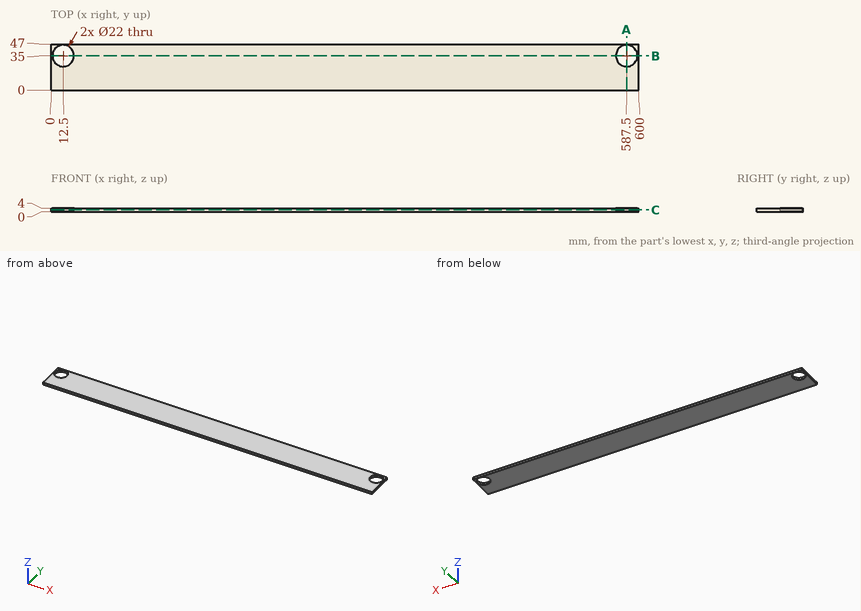
Can you work these out from the drawing? Everything is in mm from the part's minimum corner. Coordinates: 2 decimals unless noted, no trailing zeros. Loops run counter-clockwise (first coordinate to the right, second up) from the corner with the lowest first, then second, coordinate; pieces in that order, holes last.
1. Imagine slicing it at B-B, the plane y = 35. Please give me the cut outline in (x, z).
2. Imagine slicing it at A-A, the plane x = 587.5. Please give me the cut outline in (y, z), and give its area (3 significant figures).
3. Imagine slicing it at C-C, the plane z = 2.2. Please give me the cut outline in (x, y), and give its area (3 significant figures).
4. I need wall thicknesses on L1, parallel to X at y = 35.5, z = 2.5; L2, parallel to Y at x = 12.5, z = 1.4; L3, parallel to X at y = 43.5, z = 1.3. Which ranges of each line are inside material? Lowest first, please.
Taken from the geometry:
1. outline: (0, 0) - (1.5, 0) - (1.5, 4) - (0, 4) - close; (23.5, 0) - (576.5, 0) - (576.5, 4) - (23.5, 4) - close; (598.5, 0) - (600, 0) - (600, 4) - (598.5, 4) - close
2. outline: (0, 0) - (24, 0) - (24, 4) - (0, 4) - close; (46, 0) - (47, 0) - (47, 4) - (46, 4) - close
2. area: 100 mm2
3. outline: (0, 0) - (600, 0) - (600, 47) - (0, 47) - close; hole circle Ø22 at (12.5, 35); hole circle Ø22 at (587.5, 35)
3. area: 27,400 mm2
4. L1: x = 0 to 1.51, 23.49 to 576.51, 598.49 to 600
4. L2: y = 0 to 24, 46 to 47
4. L3: x = 0 to 5.52, 19.48 to 580.52, 594.48 to 600
